```python
from build123d import *

# Parameters (mm, degrees)
BOSS_EXTRUDE1_DEPTH = 5
CUT_EXTRUDE1_DEPTH  = 5


with BuildPart() as part:
    # Sketch1 → Boss-Extrude1 (new body)
    with BuildSketch(Plane(origin=(0, 0, 0), x_dir=(1, 0, 0), z_dir=(0, 1, 0))):
        Polygon((-163.000117017, 189.802822602), (-133.000117017, 189.802822602), (-133.000117017, 194.802822602), (-128.000117017, 194.802822602), (-128.000117017, 189.802822602), (-125.000117017, 189.802822602), (-125.000117017, 186.802822602), (-126.500117017, 186.802822602), (-126.500117017, 184.302822602), (-125.000117017, 184.302822602), (-125.000117017, 179.802822602), (-120.929768881, 179.802822602), (-120.929768881, 184.302822602), (-119.429768881, 184.302822602), (-119.429768881, 186.802822602), (-120.929768881, 186.802822602), (-120.929768881, 189.802822602), (-118.000117017, 189.802822602), (-118.000117017, 194.802822602), (-113.000117017, 194.802822602), (-113.000117017, 189.802822602), (-13.000117017, 189.802822602), (-13.000117017, 194.802822602), (-8.000117017, 194.802822602), (-8.000117017, 189.802822602), (-5.070465153, 189.802822602), (-5.070465153, 186.802822602), (-6.570465153, 186.802822602), (-6.570465153, 184.302822602), (-5.070465153, 184.302822602), (-5.070465153, 179.802822602), (-1.000117017, 179.802822602), (-1.000117017, 184.302822602), (0.499882983, 184.302822602), (0.499882983, 186.802822602), (-1.000117017, 186.802822602), (-1.000117017, 189.802822602), (1.999882983, 189.802822602), (1.999882983, 194.802822602), (6.999882983, 194.802822602), (6.999882983, 189.802822602), (36.999882983, 189.802822602), (36.999882983, -110.197177398), (-163.000117017, -110.197177398), align=None)
    extrude(amount=BOSS_EXTRUDE1_DEPTH)

    # Sketch2 → Cut-Extrude1 (cut)
    with BuildSketch(Plane(origin=(0, 5, 0), x_dir=(1, 0, 0), z_dir=(0, 1, 0))):
        Polygon((3.664882983, 143.66744931), (20.329882983, 114.802822602), (3.664882983, 85.938195894), (-29.665117017, 85.938195894), (-46.330117017, 114.802822602), (-29.665117017, 143.66744931), align=None)
        Polygon((-79.670117017, 114.802822602), (-96.335117017, 143.66744931), (-129.665117017, 143.66744931), (-146.330117017, 114.802822602), (-129.665117017, 85.938195894), (-96.335117017, 85.938195894), align=None)
        Polygon((-29.665117017, -64.061804106), (3.664882983, -64.061804106), (20.329882983, -35.197177398), (3.664882983, -6.33255069), (-29.665117017, -6.33255069), (-46.330117017, -35.197177398), align=None)
        Polygon((-79.670117017, -35.197177398), (-96.335117017, -64.061804106), (-129.665117017, -64.061804106), (-146.330117017, -35.197177398), (-129.665117017, -6.33255069), (-96.335117017, -6.33255069), align=None)
        Polygon((-29.670117017, 39.802822602), (-46.335117017, 68.66744931), (-79.665117017, 68.66744931), (-96.330117017, 39.802822602), (-79.665117017, 10.938195894), (-46.335117017, 10.938195894), align=None)
    extrude(amount=-CUT_EXTRUDE1_DEPTH, mode=Mode.SUBTRACT)


solid = part.part
```
Geometry: final body of the model. Coordinates: model frame, mm. Give positions to 0.01 mm unless a question says otherwise; leave off trailing zeros. Loops run counter-clockwise (first coordinate to the right, second up) from the corner with the lowest first, then second, coordinate; pieces in that order, holes last. Notation, with made-up numbers: (14.5, -28) -> (50.5, -28) arc R15 ccw to (50.5, -10) -> close; hole circle Ø5 at (2, -27.75). An arc over 180 degrees is marked (long way). Return JSON: item names as keys, results as strings.
Item 1: Section B-B, the plane z = 24. Output: boundary loops of the cut face in (x, y).
Filled in:
{"outline": "(-163, 0) -> (-139.87, 0) -> (-139.87, 5) -> (-163, 5) -> close; (-86.13, 0) -> (-39.87, 0) -> (-39.87, 5) -> (-86.13, 5) -> close; (13.87, 0) -> (37, 0) -> (37, 5) -> (13.87, 5) -> close"}
Item 2: Section C-C, the plane z = -59. Output: boundary loops of the cut face in (x, y).
Filled in:
{"outline": "(-163, 0) -> (-85.25, 0) -> (-85.25, 5) -> (-163, 5) -> close; (-40.75, 0) -> (37, 0) -> (37, 5) -> (-40.75, 5) -> close"}
Item 3: Pin query (flat end, axial travel): P1, Ø2.5, axis at x = -63, y = 3, coming from the -Z side; P2, Ø1.5, axis at y = 2, z = -192.5, coming from the +X side; P3, Ø2.5, axis at y = 3.5, z = -191.5, coming from the -X side. Return the tip coordinate at first contact, or that it passes through.
Filled in:
{"P1": "z = -189.8", "P2": "x = 7", "P3": "x = -133"}
Item 4: Section D-D, the plane y = 3.45. Count the separate pieces of the cut face and the enclosed holes in it, plus the area to 3 significant figures.
Filled in:
{"separate pieces": "1", "enclosed holes": "5", "area": "45,600 mm^2"}
Item 5: Mould query, pull axis Z, two halves, no side actions, for faces 1 (the flat face through (-62, 5, -78)), 2 (the flat face through (-138.114, 2.535, 20.967)). Classes: released by +Z, released by -Z, zero draft, split by the parting line, or undercut.
Filled in:
{"face 1": "zero draft", "face 2": "undercut"}
Item 6: Section A-A, the plane x = -55. Output: boundary loops of the cut face in (y, z).
Filled in:
{"outline": "(0, -189.8) -> (5, -189.8) -> (5, -68.67) -> (0, -68.67) -> close; (0, -10.94) -> (5, -10.94) -> (5, 110.2) -> (0, 110.2) -> close"}
Item 7: Line query: line 1 (Z direction, x = -11.5, y = 3.2); line 2 (Z direction, x = -6, y = 2.6); line 3 (Z direction, x = -23, y = 3.95). Output: solid intervals per line, ascending.
Filled in:
{"line 1": "-194.8 to -143.67, -85.94 to 6.33, 64.06 to 110.2", "line 2": "-189.8 to -186.8, -184.3 to -143.67, -85.94 to 6.33, 64.06 to 110.2", "line 3": "-189.8 to -143.67, -85.94 to 6.33, 64.06 to 110.2"}
